Could you check a few things on this model? Use its own coordinates, in mm. Face numbers are marked on the shaded views. A direction names the side the tool comes from. Coordinates: 2 decimals unless noted, no trailing zeros. Loops run counter-clockwise (first coordinate to the right, second up) from the corner with the lowest first, then second, coordinate; pieces in that order, holes last.
1) If I drill on line 1 along X through (y, z) = (-116, 31.5); line 2 along X through (y, z) = (-144, 26.5); line 3 along Z through (x, y) = (-50.5, -127), over which ranges is the centre line in solid material (lowest first)?
2) For the marked faces 1 and 2, which set-ups out of +Z, -Z, +X, -X, +Y, -Y let a thin tool reach every point of the face, with its end or its side?
3) Imagine slicing it at B-B on y = -17. Please give me the cut outline in (x, z).
4) Imagine slicing it at C-C on x = -56. Please give me the cut outline in (y, z), plus the area to 3 significant figures.
5) Will these pins go through, and if not, where does the flat tip stop? P1, Ø2, axis at x = -40, y = -79.5, coming from the -Z side; P2, Ø12, axis at x = -56, y = -75, coming from the -Z side; P3, Ø12, axis at x = 11, z = 27.5, coming from the -Y side.
6) Thinking about a two-plate mould opening in Z: for the marked faces 3, 4 and 5, which applies, released by +Z, released by -Z, zero draft, split by the parting line, or undercut?
7) Imagine slicing it at A-A on z = 36. Please give me the cut outline in (x, y), plus the area to 3 significant figures.
8) Imagine slicing it at D-D on z = 9.5. Please give me the cut outline in (x, y), plus the area to 3 significant figures.
```python
from build123d import *

# Parameters (mm, degrees)
F1_DEPTH = 150


with BuildPart() as f1:
    # F0 (on Front) → F1 (new body)
    with BuildSketch(Plane.XZ):
        Polygon((-0.930744, 18.957937), (9.735235, -2.667266), (89.069256, 21.56038), (89.069256, 60.261399), (-0.930744, 60.261399), (-90.930744, 60.261399), (-90.930744, 21.56038), (-11.596724, -2.667266), align=None)
        Polygon((84.069252, 25.261401), (12.339529, 3.356015), (-0.930744, 30.261407), (-14.201018, 3.356015), (-85.930741, 25.261401), (-85.930741, 55.261395), (-0.930744, 55.261395), (84.069252, 55.261395), align=None, mode=Mode.SUBTRACT)
    extrude(amount=F1_DEPTH)


solid = f1.part
```
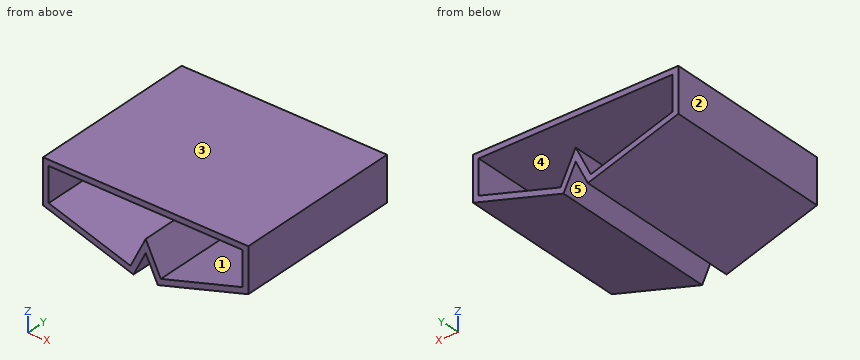
Filled in:
1. line 1: x = -90.93 to -85.93, 84.07 to 89.07
1. line 2: x = -90.93 to -85.93, -2.79 to 0.92, 84.07 to 89.07
1. line 3: z = 9.21 to 14.44, 55.26 to 60.26
2. face 1: +Y, -Y
2. face 2: +Z, -Z, -X, +Y, -Y
3. outline: (-90.93, 21.56) - (-11.6, -2.67) - (-0.93, 18.96) - (9.74, -2.67) - (89.07, 21.56) - (89.07, 60.26) - (-90.93, 60.26) - close; hole (-85.93, 25.26) - (-14.2, 3.36) - (-0.93, 30.26) - (12.34, 3.36) - (84.07, 25.26) - (84.07, 55.26) - (-85.93, 55.26) - close
4. outline: (-150, 10.89) - (0, 10.89) - (0, 16.12) - (-150, 16.12) - close; (-150, 55.26) - (0, 55.26) - (0, 60.26) - (-150, 60.26) - close
4. area: 1,530 mm2
5. P1: stops at z = 5.7
5. P2: stops at z = 9.06
5. P3: passes through
6. face 3: released by +Z
6. face 4: undercut
6. face 5: released by -Z
7. outline: (-90.93, -150) - (-85.93, -150) - (-85.93, 0) - (-90.93, 0) - close; (84.07, -150) - (89.07, -150) - (89.07, 0) - (84.07, 0) - close
7. area: 1,500 mm2
8. outline: (-51.44, -150) - (-34.32, -150) - (-34.32, 0) - (-51.44, 0) - close; (-11.17, -150) - (-5.6, -150) - (-5.6, 0) - (-11.17, 0) - close; (3.73, -150) - (9.31, -150) - (9.31, 0) - (3.73, 0) - close; (32.46, -150) - (49.58, -150) - (49.58, 0) - (32.46, 0) - close
8. area: 6,810 mm2
